For this review, take the finished solid that the model builds, in its own axes (mm). A direction names the side the tool comes from. Round coordinates to 2 decimals unless told otherwise and drop trailing zeros. Order: outer loops, then holes, each group sorted by start corner. A loop starts at its lowest first (then second) coordinate and runs counter-clockwise, first axis right, second up. Notation, with made-up numbers: M -25.75,54.25 L -8.75,54.25 A24 cw -8.75,92.25 Z; hole C 74.25,-8.5 d4. An arc over 180 degrees is marked long. Answer as a JSON object with one key per item and string values.
Autodesk Fusion 360 part; units mm, degrees
sketch "Boceto1" plane through (0, 0, 0) normal (0, 0, 1) x (1, 0, 0)
  line L0 (4.725, 2.765) -> (4.725, -5.635)
  line L1 (4.725, -8.235) -> (-4.725, -8.235)
  line L2 (-4.725, -8.235) -> (-4.725, 2.765)
  line L3 (-6.225, 4.265) -> (6.225, 4.265)
  line L4 (6.225, 4.265) -> (6.225, -9.735)
  line L5 (6.225, -9.735) -> (-6.225, -9.735)
  line L6 (-6.225, -9.735) -> (-6.225, 4.265)
  line L7 (2.585, -4.215) -> (2.585, -6.945)
  line L8 (2.585, -6.945) -> (-3.075, -6.945)
  line L9 (-3.075, -6.945) -> (-3.075, -4.215)
  line L10 (-1.61, -4.215) -> (-1.61, 1.765)
  line L11 (1.61, 1.765) -> (1.61, -4.215)
  line L12 (-3.075, -4.215) -> (-1.61, -4.215)
  line L13 (1.61, -4.215) -> (2.585, -4.215)
  line L14 (-4.725, 2.765) -> (-4.725, 4.265)
  line L15 (4.725, 4.265) -> (4.725, 2.765)
  line L16 (4.725, -5.635) -> (6.225, -5.635)
  line L17 (4.725, -8.235) -> (6.225, -8.235)
  line L18 (-1.61, 1.765) -> (1.61, 1.765)
  dimension "d1" = 9.45
  dimension "d2" = 4.725
  dimension "d3" = 1.5
  dimension "d4" = 1.5
  dimension "d5" = 1.5
  dimension "d6" = 1.5
  dimension "d9" = 8.235
  dimension "d10" = 5.66
  dimension "d11" = 2.73
  dimension "d12" = 1.29
  dimension "d13" = 1.65
  dimension "d21" = 10
  dimension "d22" = 12.5
  dimension "d27" = 2.6
  dimension "d32" = 3.115
  dimension "d33" = 3.115
extrude "Extruir5" add sketch "Boceto1" against normal blind 1.5 contours L0 L1 L2 L3 L4 L14 L15 L16 L17
extrude "Extruir6" add sketch "Boceto1" against normal blind 6.5 contours L0 L3 L4 L15 L16 | L1 L2 L3 L4 L5 L6 L14 L17
extrude "Extruir7" cut 1 faces at (-4.725, -4.0683, -3.1667) along direction (-1, 0, 0) blind 0.2
extrude "Extruir8" cut 1 faces at (4.725, 0.965, -3.1667) along direction (1, 0, 0) blind 0.2
equation "d2 = d1 / 2"
equation "d4 = d3"
equation "d5 = d3"
equation "d6 = d3"
equation "d9 = d7 / 2"
equation "d22 = d21 + d3 + 1 mm"
equation "d28 = -d3"
equation "d30 = -( d3 + 5 mm )"
equation "d32 = d1 / 2 - ( ( 3.22 / 2 ) * 1 mm )"
equation "d33 = d32"
1) Add section C-C on z = -1.25. State the section outline as (x, y) points (3 decimals).
Geometry check:
{"outline": "M -6.225,-9.735 L 6.225,-9.735 L 6.225,4.265 L -6.225,4.265 Z; hole M -3.075,-6.945 L 2.585,-6.945 L 2.585,-4.215 L 1.61,-4.215 L 1.61,1.765 L -1.61,1.765 L -1.61,-4.215 L -3.075,-4.215 Z"}
2) Mouldability with a two-part tool opening along Y and no side actions: class faces 6 (the flat face through (-2, -4.215, -1)), 7 (the flat face through (0, -9.735, -3)), 8 (the flat face through (6.225, -1, -3)) as +Y half, -Y half, draft (parallel to the pull), parting line (faces both ways), or undercut.
Geometry check:
{"face 6": "undercut", "face 7": "-Y half", "face 8": "draft"}
3) Insertion check: P1, Ø5, axis at x = 5, y = -7.5, coming from the +Z side; P2, Ø1, axis at y = -7.5, z = -4, coming from the +X side (3 decimals); P3, Ø3.5, axis at x = -1.5, y = 1, coming from the -Z side; P4, Ø3, axis at x = 1, z = -5.5, coming from the +Y side (3 decimals). Each pin has a flat end and moves straight along its axis. Give the tip position at first contact, or say it passes through.
Geometry check:
{"P1": "stops at z = 0", "P2": "stops at x = -4.925", "P3": "stops at z = -1.5", "P4": "stops at y = -8.235"}
4) Machinability: for faces 1 (the flat face through (-4.925, -2, -4)), 2 (the flat face through (-1.61, -1, -1)), 3 (the flat face through (-6.225, -3, -3)), 4 (the flat face through (6, -5.635, -4)), 5 (the flat face through (-5.1, -5.8, -6.5)), which of the approach directions +Z, -Z, +X, -X, +Y, -Y give a long, thin tool a straight path to every point of the face, cutting with its end or side? Answer none if there is none.
Geometry check:
{"face 1": "-Z, +Y", "face 2": "+Z, -Z", "face 3": "+Z, -Z, -X, +Y, -Y", "face 4": "-Z, +X", "face 5": "-Z, +X, -X, +Y, -Y"}
5) Add section B-B on x = -2.5. State the section outline as (y, z) points (3 decimals).
Geometry check:
{"outline": "M -9.735,-6.5 L -8.235,-6.5 L -8.235,-1.5 L -6.945,-1.5 L -6.945,0 L -9.735,0 Z; M -4.215,-1.5 L 4.265,-1.5 L 4.265,0 L -4.215,0 Z"}
6) Add section D-D on y = 2.75. State the section outline as (x, z) points (3 decimals).
Geometry check:
{"outline": "M -6.225,-6.5 L -4.925,-6.5 L -4.925,-1.5 L 4.925,-1.5 L 4.925,-6.5 L 6.225,-6.5 L 6.225,0 L -6.225,0 Z"}
7) For L1, parallel to Y at x = -0.25, z = -0.5 (3 decimals); L2, parallel to X at y = -4.25, z = -3.25 (3 decimals); L3, parallel to Y at x = 5.5, z = -4 (3 decimals), list the stretches that pass through material, from the lowest coordinate up.
Geometry check:
{"L1": "y = -9.735 to -6.945, 1.765 to 4.265", "L2": "x = -6.225 to -4.925, 4.925 to 6.225", "L3": "y = -9.735 to -8.235, -5.635 to 4.265"}
8) Add section A-A on y = -6. State the section outline as (x, z) points (3 decimals), and give its area (3 significant figures).
Geometry check:
{"outline": "M -6.225,-6.5 L -4.925,-6.5 L -4.925,-1.5 L -3.075,-1.5 L -3.075,0 L -6.225,0 Z; M 2.585,-1.5 L 6.225,-1.5 L 6.225,0 L 2.585,0 Z", "area": "16.7 mm²"}
